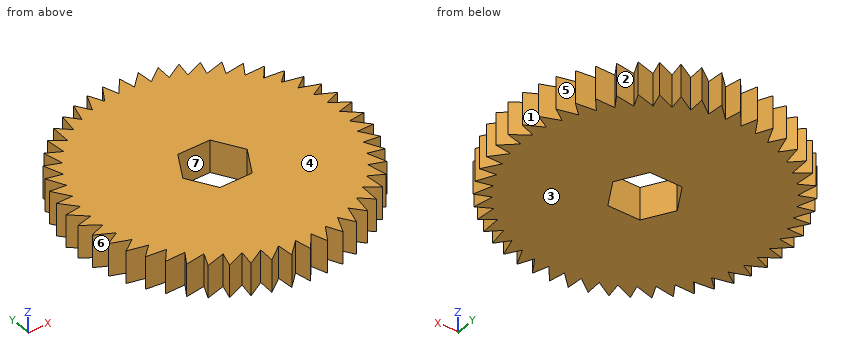
from build123d import *

# Parameters (mm, degrees)
SCHIZZO1_R                    = 42.70134189
ESTRUSIONE_ESTRUSIONE2_DEPTH  = 5
TAGLIO_ESTRUSIONE4_DEPTH      = 62.21118524
TAGLIO_ESTRUSIONE4_DEPTH_BACK = 62.21118524
TAGLIO_ESTRUSIONE5_DEPTH      = 62.21118524
RIPETIZIONECIRCOLARE1_COUNT   = 50


with BuildPart() as part:
    # Schizzo1 → Estrusione-Estrusione2 (new, symmetric)
    with BuildSketch(Plane.XY):
        Circle(SCHIZZO1_R)
    extrude(amount=ESTRUSIONE_ESTRUSIONE2_DEPTH, both=True)

    # Schizzo6 → Taglio-Estrusione4 (cut, two sides: drawn at the far end of the back side and taken through both)
    with BuildSketch(Plane.XY.offset(5).offset(-TAGLIO_ESTRUSIONE4_DEPTH_BACK)):
        Polygon((10, 0), (5, 8.660254038), (-5, 8.660254038), (-10, 0), (-5, -8.660254038), (5, -8.660254038), align=None)
    extrude(amount=TAGLIO_ESTRUSIONE4_DEPTH + TAGLIO_ESTRUSIONE4_DEPTH_BACK, mode=Mode.SUBTRACT)

    # Schizzo7 → Taglio-Estrusione5 (cut, through all)
    with BuildSketch(Plane.XY.offset(5)):
        Polygon((-9.417976615, 44.546082505), (-5.993285857, 37.316179794), (-1.087643203, 45.316179794), align=None)
    taglio_estrusione5 = extrude(amount=-TAGLIO_ESTRUSIONE5_DEPTH, mode=Mode.SUBTRACT)

    # RipetizioneCircolare1: Taglio-Estrusione5 ×50 about axis
    ripetizionecircolare1_axis = Axis((0, 0, 0), (0, 0, 1))
    for i in range(1, RIPETIZIONECIRCOLARE1_COUNT):
        add(taglio_estrusione5.rotate(ripetizionecircolare1_axis, i * 360 / RIPETIZIONECIRCOLARE1_COUNT), mode=Mode.SUBTRACT)


solid = part.part
Design review of the part built by this model. Coordinates are the model's own, in mm. Face numbers are marked on the shaded views. A direction names the side the tool comes from. Round coordinates to 2 decimals unless told otherwise and drop trailing zeros.
Item 1: Wall thickness on L1, parallel to X at y = 35.5, z = 1.75; L2, parallel to Y at x = 7, z = -4; L3, parallel to Y at x = -5.5, z = -4: over which ranges is each line inside the solid? List them lowest first.
Item 2: For the marked faces 4, 5, 6 and 7, list the 3-axis set-ups (+Z, -Z, +X, -X, +Y, -Y) from which the entire face can be reached by the end or side of a thin tool; tool diameter is ignored.
Item 3: For pin 1 Ø1 at (y, z) = (17, -1.5) entering from -X; pin 2 Ø5 at (x, z) = (-1, -0.5) entering from -Y; pin 3 Ø5 at (x, z) = (27, -1.5) entering from +Y, all flat-tipped, find the tip position at first contact; note any pin that passes through.
Item 4: Draft analysis for pull direction X (two halves, no side actions). For the marked faces 1, 2 and 3, state which applies: released by +X, released by -X, zero draft, split by the parting line, or undercut.
Check values:
1. L1: x = -22.96 to -22.53, -18.78 to -15.79, -14.82 to 17.42, 21.4 to 22.53
1. L2: y = -39.44 to -5.2, 5.2 to 41.05
1. L3: y = -39.6 to -7.79, 7.79 to 38.12
2. face 4: +Z, +X, -X, +Y, -Y
2. face 5: +Z, -Z, +X
2. face 6: +Z, -Z, -X
2. face 7: +Z, -Z
3. pin 1: stops at x = -35.97
3. pin 2: stops at y = -42.51
3. pin 3: stops at y = 32.91
4. face 1: released by +X
4. face 2: undercut
4. face 3: zero draft
